Model file for the job. Use its own axes, mm. A direction names the side the tool comes from. Coordinates: 2 decimals unless noted, no trailing zeros. Loops run counter-clockwise (first coordinate to the right, second up) from the corner with the lowest first, then second, coordinate; pieces in that order, holes last. Notation, with made-up numbers: (-4.75, -5) -> (45.25, -5) arc R27 ccw to (45.25, 15) -> close; hole circle Ø5 at (-14.5, -36). An arc over 180 degrees is marked (long way). Use one line per item in the form item = value.
```python
from build123d import *

# Parameters (mm, degrees)
SKETCH1_R            = 1.15
BOSS_EXTRUDE1_DEPTH  = 1
BOSS_EXTRUDE2_DEPTH  = 12
BOSS_EXTRUDE3_DEPTH  = 12
SKETCH6_W            = 6.853919328
SKETCH6_H            = 5
BOSS_EXTRUDE4_DEPTH  = 10
MIRROR2_START        = -11
MIRROR2_OUTLINE_R    = 1.15
MIRROR2_DEPTH        = 1
MIRROR2_START_2      = -10
MIRROR2_2_DEPTH      = 11
SKETCH7_W            = 11.75623079
SKETCH7_H            = 5.445993007
CUT_EXTRUDE1_DEPTH   = 22
SKETCH15_W           = 6.853919328
SKETCH15_H           = 5
BOSS_EXTRUDE8_DEPTH  = 6.873966159
CUT_EXTRUDE6_DEPTH   = 10
BOSS_EXTRUDE9_DEPTH  = 3.5
SKETCH19_R           = 1.15
CUT_EXTRUDE2_DEPTH   = 20
BOSS_EXTRUDE10_DEPTH = 1
BOSS_EXTRUDE11_START = 3
SKETCH27_R           = 1.15
BOSS_EXTRUDE11_DEPTH = 3
SKETCH28_W           = 13.273966158
SKETCH28_H           = 6
CUT_EXTRUDE7_DEPTH   = 13
SKETCH29_W           = 6.853919328
SKETCH29_H           = 6.073966158
SKETCH29_R           = 1.15
BOSS_EXTRUDE12_DEPTH = 13
BOSS_EXTRUDE13_DEPTH = 4


with BuildPart() as part:
    # Sketch1 → Boss-Extrude1 (new body)
    with BuildSketch(Plane(origin=(0, 0, 0), x_dir=(1, 0, 0), z_dir=(0, 1, 0))):
        Polygon((-6.046966624, 49.693438145), (-5.709264166, 46.7123956), (-3.10834847, 44.45145408), (-2.33209021, 44.498932069), (-0.026100804, 47.059992762), (0.026100804, 47.059992762), (2.33209021, 44.498932069), (3.10834847, 44.45145408), (5.709264166, 46.7123956), (6.046966624, 49.693438145), (3.66640026, 52.431966482), (2.75077786, 52.487968347), (0.054213226, 50.059970644), (-0.054213226, 50.059970644), (-2.75077786, 52.487968347), (-3.66640026, 52.431966482), align=None)
        with Locations(Location((-3.086614159, 50.465695408, 0), (0, 0, 270))):
            Circle(SKETCH1_R, mode=Mode.SUBTRACT)
        with Locations(Location((3.086614159, 50.465695408, 0), (0, 0, 270))):
            Circle(SKETCH1_R, mode=Mode.SUBTRACT)
        with Locations(Location((2.842648162, 46.476886618, 0), (0, 0, 270))):
            Circle(SKETCH1_R, mode=Mode.SUBTRACT)
        with Locations(Location((-2.842648162, 46.476886618, 0), (0, 0, 270))):
            Circle(SKETCH1_R, mode=Mode.SUBTRACT)
    boss_extrude1 = extrude(amount=BOSS_EXTRUDE1_DEPTH)

    # Sketch2 → Boss-Extrude2 (add)
    with BuildSketch(Plane(origin=(0, 1, 0), x_dir=(1, 0, 0), z_dir=(0, 1, 0))):
        Polygon((-3.66640026, 52.431966482), (-2.75077786, 52.487968347), (-2.799616692, 53.286476185), (-3.715239092, 53.23047432), align=None)
        Polygon((2.75077786, 52.487968347), (3.66640026, 52.431966482), (3.715239092, 53.23047432), (2.799616692, 53.286476185), align=None)
    extrude(amount=-BOSS_EXTRUDE2_DEPTH)

    # Mirror1: Boss-Extrude1 across plane
    add(boss_extrude1.mirror(Plane.ZX.offset(-5)))

    # Sketch3 → Boss-Extrude3 (add)
    with BuildSketch(Plane(origin=(0, 1, 0), x_dir=(1, 0, 0), z_dir=(0, 1, 0))):
        Polygon((2.33209021, 44.498932069), (3.10834847, 44.45145408), (3.059509638, 43.652946241), (2.283251379, 43.70042423), align=None)
        Polygon((-2.33209021, 44.498932069), (-3.10834847, 44.45145408), (-3.059509638, 43.652946241), (-2.283251379, 43.70042423), align=None)
    extrude(amount=-BOSS_EXTRUDE3_DEPTH)

    # Sketch6 → Boss-Extrude4 (add)
    with BuildSketch(Plane(origin=(0, 0, -53.059970644), x_dir=(-1, 0, 0), z_dir=(0, 0, -1))):
        with Locations((0, -5)):
            Rectangle(SKETCH6_W, SKETCH6_H)
    extrude(amount=BOSS_EXTRUDE4_DEPTH)



with BuildPart() as body_2:
    # Mirror2: read off the stored shape, not the designer's step
    # Mirror2 outline → Mirror2 (new body)
    with BuildSketch(Plane(origin=(0, 0, 0), x_dir=(1, 0, 0), z_dir=(0, 1, 0)).offset(MIRROR2_START)):
        Polygon((-3.715239092, 62.889466969), (-2.799616692, 62.833465104), (-2.75077786, 63.631972942), (-0.054213226, 66.059970644), (0.054213226, 66.059970644), (2.75077786, 63.631972942), (2.799616692, 62.833465104), (3.715239092, 62.889466969), (3.66640026, 63.687974807), (6.046966624, 66.426503144), (5.709264166, 69.407545689), (3.10834847, 71.668487209), (3.059509638, 72.466995048), (2.283251379, 72.419517059), (2.33209021, 71.62100922), (0.026100804, 69.059948527), (-0.026100804, 69.059948527), (-2.33209021, 71.62100922), (-2.283251379, 72.419517059), (-3.059509638, 72.466995048), (-3.10834847, 71.668487209), (-5.709264166, 69.407545689), (-6.046966624, 66.426503144), (-3.66640026, 63.687974807), align=None)
        with Locations((2.842648162, 69.643054671)):
            Circle(MIRROR2_OUTLINE_R, mode=Mode.SUBTRACT)
        with Locations((-3.086614159, 65.654245881)):
            Circle(MIRROR2_OUTLINE_R, mode=Mode.SUBTRACT)
        with Locations((3.086614159, 65.654245881)):
            Circle(MIRROR2_OUTLINE_R, mode=Mode.SUBTRACT)
        with Locations((-2.842648162, 69.643054671)):
            Circle(MIRROR2_OUTLINE_R, mode=Mode.SUBTRACT)
    mirror2 = extrude(amount=MIRROR2_DEPTH)


with BuildPart() as part_1:
    add(part.part)

    add(body_2.part)  # Mirror2 2 merges body 2
    # Mirror2 2 outline → Mirror2 2 (add)
    with BuildSketch(Plane(origin=(0, 0, 0), x_dir=(1, 0, 0), z_dir=(0, 1, 0)).offset(MIRROR2_START_2)):
        Polygon((-3.715239092, 62.889466969), (-2.799616692, 62.833465104), (-2.75077786, 63.631972942), (-3.66640026, 63.687974807), align=None)
        Polygon((3.66640026, 63.687974807), (2.75077786, 63.631972942), (2.799616692, 62.833465104), (3.715239092, 62.889466969), align=None)
        Polygon((-3.059509638, 72.466995048), (-3.10834847, 71.668487209), (-2.33209021, 71.62100922), (-2.283251379, 72.419517059), align=None)
        Polygon((2.33209021, 71.62100922), (3.10834847, 71.668487209), (3.059509638, 72.466995048), (2.283251379, 72.419517059), align=None)
    mirror2_2 = extrude(amount=MIRROR2_2_DEPTH)

    # Mirror3: Mirror2, Mirror2 2 across plane
    add(mirror2.mirror(Plane.ZX.offset(-5)))
    add(mirror2_2.mirror(Plane.ZX.offset(-5)))

    # Sketch7 → Cut-Extrude1 (cut)
    with BuildSketch(Plane.XZ.offset(11)):
        with Locations((0, -45.479920369)):
            Rectangle(SKETCH7_W, SKETCH7_H)
    cut_extrude1 = extrude(amount=-CUT_EXTRUDE1_DEPTH, mode=Mode.SUBTRACT)

    # Mirror4: Cut-Extrude1 across plane
    add(cut_extrude1.mirror(Plane.XY.offset(-58.059970644)), mode=Mode.SUBTRACT)


with BuildPart() as body_2_2:
    # Split1: the piece on the far side of the plane
    add(part_1.part)
    split(bisect_by=Plane.XY.offset(-58.059970644), keep=Keep.BOTTOM)


with BuildPart() as part_2:
    add(part_1.part)

    # Split1
    split(bisect_by=Plane.XY.offset(-58.059970644), keep=Keep.TOP)


with BuildPart() as part_3:
    # Body-Move/Copy1: moved
    add(part_2.part.moved(Location((0, 0, 6.873966159))))


with BuildPart() as part_4:
    # Body-Move/Copy2: moved
    add(part_3.part.moved(Location((20.680073688, 0, 0))))


with BuildPart() as part_5:
    # Body-Move/Copy4: read off the stored shape, not the designer's step
    # Body-Move/Copy4: moved
    add(part_4.part.moved(Location((-20.6800737, 0, 0))))


    add(body_2_2.part)  # Boss-Extrude8 merges body 2 2
    # Sketch15 → Boss-Extrude8 (add)
    with BuildSketch(Plane.XY.offset(-58.059970644)):
        with Locations((0, -5)):
            Rectangle(SKETCH15_W, SKETCH15_H)
    extrude(amount=BOSS_EXTRUDE8_DEPTH)

    # Sketch24 → Cut-Extrude6 (cut)
    with BuildSketch(Plane(origin=(0, -2.5, 0), x_dir=(1, 0, 0), z_dir=(0, 1, 0))):
        Polygon((-3.426959664, 61.259970644), (-3.426959664, 57.659970644), (-0.3, 59.459970644), align=None)
        Polygon((3.426959664, 61.259970644), (0.3, 59.459970644), (3.426959664, 57.659970644), align=None)
    cut_extrude6 = extrude(amount=-CUT_EXTRUDE6_DEPTH, mode=Mode.SUBTRACT)

    # Mirror8: Cut-Extrude6 across plane
    add(cut_extrude6.mirror(Plane.XY.offset(-54.622987565)), mode=Mode.SUBTRACT)

    # Sketch25 → Boss-Extrude9 (add)
    with BuildSketch(Plane(origin=(0, -2.5, 0), x_dir=(1, 0, 0), z_dir=(0, 1, 0))):
        Polygon((-3.426959664, 63.059970644), (-3.426959664, 61.259970644), (-0.3, 59.459970644), (-3.426959664, 57.659970644), (-3.426959664, 51.586004486), (-0.3, 49.786004486), (-3.426959664, 47.986004486), (-3.426959664, 46.186004486), (3.426959664, 46.186004486), (3.426959664, 47.986004486), (0.3, 49.786004486), (3.426959664, 51.586004486), (3.426959664, 57.659970644), (0.3, 59.459970644), (3.426959664, 61.259970644), (3.426959664, 63.059970644), align=None)
    boss_extrude9 = extrude(amount=BOSS_EXTRUDE9_DEPTH)

    # Mirror10: Boss-Extrude9 across plane
    add(boss_extrude9.mirror(Plane.ZX.offset(-5)))

    # Sketch19 → Cut-Extrude2 (cut)
    with BuildSketch(Plane(origin=(0, 1, 0), x_dir=(1, 0, 0), z_dir=(0, 1, 0))):
        with Locations(Location((0, 54.622987565, 0), (0, 0, 270))):
            Circle(SKETCH19_R)
    extrude(amount=-CUT_EXTRUDE2_DEPTH, mode=Mode.SUBTRACT)

    # Sketch26 → Boss-Extrude10 (add)
    with BuildSketch(Plane(origin=(0, 1, 0), x_dir=(1, 0, 0), z_dir=(0, 1, 0))):
        Polygon((-0.054213226, 66.059970644), (0.054213226, 66.059970644), (2.75077786, 63.631972942), (2.785763019, 63.059970644), (-2.785763019, 63.059970644), (-2.75077786, 63.631972942), align=None)
        Polygon((-2.785763019, 46.186004486), (2.785763019, 46.186004486), (2.75077786, 45.614002188), (0.054213226, 43.186004486), (-0.054213226, 43.186004486), (-2.75077786, 45.614002188), align=None)
    boss_extrude10 = extrude(amount=-BOSS_EXTRUDE10_DEPTH)

    # Mirror11: Boss-Extrude10 across plane
    add(boss_extrude10.mirror(Plane.ZX.offset(-5)))

    # Sketch27 → Boss-Extrude11 (add)
    with BuildSketch(Plane(origin=(0, 1, 0), x_dir=(1, 0, 0), z_dir=(0, 1, 0)).offset(BOSS_EXTRUDE11_START)):
        Polygon((-5.878115395, 67.917024417), (-6.046966624, 66.426503144), (-3.66640026, 63.687974807), (-3.715239092, 62.889466969), (-3.426959664, 62.871835043), (-3.426959664, 61.259970644), (-0.3, 59.459970644), (-3.426959664, 57.659970644), (-3.426959664, 51.586004486), (-0.3, 49.786004486), (-3.426959664, 47.986004486), (-3.426959664, 46.374140087), (-3.715239092, 46.356508162), (-3.66640026, 45.558000323), (-6.046966624, 42.819471986), (-5.878115395, 41.328950714), (5.878115395, 41.328950714), (6.046966624, 42.819471986), (3.66640026, 45.558000323), (3.715239092, 46.356508162), (3.426959664, 46.374140087), (3.426959664, 47.986004486), (0.3, 49.786004486), (3.426959664, 51.586004486), (3.426959664, 57.659970644), (0.3, 59.459970644), (3.426959664, 61.259970644), (3.426959664, 62.871835043), (3.715239092, 62.889466969), (3.66640026, 63.687974807), (6.046966624, 66.426503144), (5.878115395, 67.917024417), align=None)
        with Locations(Location((-3.086614159, 65.654245881, 0), (0, 0, 90))):
            Circle(SKETCH27_R, mode=Mode.SUBTRACT)
        with Locations(Location((3.086614159, 65.654245881, 0), (0, 0, 90))):
            Circle(SKETCH27_R, mode=Mode.SUBTRACT)
        with Locations(Location((0, 54.622987565, 0), (0, 0, 270))):
            Circle(SKETCH27_R, mode=Mode.SUBTRACT)
        with Locations(Location((-3.086614159, 43.59172925, 0), (0, 0, 270))):
            Circle(SKETCH27_R, mode=Mode.SUBTRACT)
        with Locations(Location((3.086614159, 43.59172925, 0), (0, 0, 270))):
            Circle(SKETCH27_R, mode=Mode.SUBTRACT)
    boss_extrude11 = extrude(amount=-BOSS_EXTRUDE11_DEPTH)

    # Mirror12: Boss-Extrude11 across plane
    add(boss_extrude11.mirror(Plane.ZX.offset(-5)))

    # Sketch28 → Cut-Extrude7 (cut)
    with BuildSketch(Plane.ZY.offset(3.426959664)):
        with Locations((-54.622987565, -5)):
            Rectangle(SKETCH28_W, SKETCH28_H)
    extrude(amount=-CUT_EXTRUDE7_DEPTH, mode=Mode.SUBTRACT)

    # Sketch29 → Boss-Extrude12 (add)
    with BuildSketch(Plane(origin=(0, 4, 0), x_dir=(1, 0, 0), z_dir=(0, 1, 0))):
        with Locations((0, 54.622987565)):
            Rectangle(SKETCH29_W, SKETCH29_H)
        with Locations(Location((0, 54.622987565, 0), (0, 0, 270))):
            Circle(SKETCH29_R, mode=Mode.SUBTRACT)
    extrude(amount=-BOSS_EXTRUDE12_DEPTH)

    # Sketch30 → Boss-Extrude13 (add)
    with BuildSketch(Plane(origin=(0, 4, 0), x_dir=(1, 0, 0), z_dir=(0, 1, 0))):
        Polygon((3.426959664, 61.259970644), (6.046966624, 66.426503144), (3.66640026, 63.687974807), (3.715239092, 62.889466969), (3.426959664, 62.871835043), align=None)
        Polygon((-6.046966624, 66.426503144), (-3.66640026, 63.687974807), (-3.715239092, 62.889466969), (-3.426959664, 62.871835043), (-3.426959664, 61.259970644), align=None)
        Polygon((3.426959664, 47.986004486), (3.426959664, 46.374140087), (3.715239092, 46.356508162), (3.66640026, 45.558000323), (6.046966624, 42.819471986), align=None)
        Polygon((-3.426959664, 47.986004486), (-3.426959664, 46.374140087), (-3.715239092, 46.356508162), (-3.66640026, 45.558000323), (-6.046966624, 42.819471986), align=None)
    boss_extrude13 = extrude(amount=-BOSS_EXTRUDE13_DEPTH)

    # Mirror13: Boss-Extrude13 across plane
    add(boss_extrude13.mirror(Plane.ZX.offset(-5)))


solid = part_5.part
```
Q1. Band-saw the part on B-B, the plane y = -3. State how many separate pieces and enclosed holes the cut face has, and give its area (3 significant figures).
Result:
separate_pieces = 3
enclosed_holes = 1
area = 64.6 mm2
Q2. Pin check, flat tips, straight feed: pin 1 Ø2 at (y, z) = (-6, -46.5) entering from +X; pin 2 Ø5 at (x, y) = (0, -3.5) entering from +Z; pin 3 Ø1.3 at (y, z) = (-7, -62) entering from +X; pin 4 Ø1.8 at (x, z) = (3.09, -43.59) entering from +Y. Stop position of each tip, or through.
Result:
pin_1 = 3.72
pin_2 = -46.19
pin_3 = 3.43
pin_4 = through
Q3. Mould opens along Y. For faces 1 (the face through (-3.427, -5, -62)), 2 (the face through (0, -12, -67.917)) say: released by +Y, released by -Y, zero draft, split by the parting line, or undercut.
Result:
face_1 = undercut
face_2 = zero draft
Q4. Band-saw the part on C-C, the plane z = -44.25. Write the cut outline in (x, y).
Result:
outline = (-5.32, -14) -> (-4.03, -14) -> (-4.03, -10) -> (-5.32, -10) -> close; (-5.32, 0) -> (-4.03, 0) -> (-4.03, 4) -> (-5.32, 4) -> close; (-2.14, -14) -> (2.14, -14) -> (2.14, -10) -> (-2.14, -10) -> close; (-2.14, 0) -> (2.14, 0) -> (2.14, 4) -> (-2.14, 4) -> close; (4.03, -14) -> (5.32, -14) -> (5.32, -10) -> (4.03, -10) -> close; (4.03, 0) -> (5.32, 0) -> (5.32, 4) -> (4.03, 4) -> close
Q5. Band-saw the part on D-D, the plane z = -54.25. Write the cut outline in (x, y).
Result:
outline = (-3.43, -14) -> (-1.09, -14) -> (-1.09, 4) -> (-3.43, 4) -> close; (1.09, -14) -> (3.43, -14) -> (3.43, 4) -> (1.09, 4) -> close
Q6. Wall check: line 1 along Z through (x, y) = (2.25, -7.5); line 2 along Y through (x, z) = (-4, -44.5); line 3 along Z through (x, y) = (-0.5, -12.5). Give the ranges that are in metal, low to high.
Result:
line_1 = -63.06 to -61.26, -57.66 to -51.59, -47.99 to -46.19
line_2 = -14 to -10, 0 to 4
line_3 = -67.92 to -59.58, -59.34 to -55.66, -53.59 to -49.9, -49.67 to -41.33
Q7. Which spindle directions (+Z, -Z, +X, -X, +Y, -Y) get a long thin tool onto all of the face, cutting with end or side? Do faces 3 (the face through (1.842, 0.958, -50.673)), 4 (the face through (0, -5, -47.986)), 5 (the face through (-1.885, 0.958, -60.373)). Say none if no direction does.
Result:
face_3 = +X, +Y, -Y
face_4 = +X, -X
face_5 = -X, +Y, -Y
Q8. Band-saw the part on A-A, the plane x = 0. Write the cut outline in (y, z), and give its area (3 significant figures).
Result:
outline = (-14, -67.92) -> (-10, -67.92) -> (-10, -63.06) -> (0, -63.06) -> (0, -67.92) -> (4, -67.92) -> (4, -55.77) -> (-14, -55.77) -> close; (-14, -53.47) -> (4, -53.47) -> (4, -41.33) -> (0, -41.33) -> (0, -46.19) -> (-10, -46.19) -> (-10, -41.33) -> (-14, -41.33) -> close; hole (-8, -61.26) -> (-2, -61.26) -> (-2, -57.66) -> (-8, -57.66) -> close; hole (-8, -51.59) -> (-2, -51.59) -> (-2, -47.99) -> (-8, -47.99) -> close
area = 297 mm2
